```python
from build123d import *

# Parameters (mm, degrees)
F0_W     = 30
F0_H     = 10
F1_DEPTH = 44
F2_R     = 3
F3_R     = 3
F5_START = 44
F4_R     = 2.75
F5_DEPTH = 18
F7_R     = 2.75
F8_ANGLE = 180
F10_W    = 6.5
F10_H    = 4
F12_SIZE = 1
F13_SIZE = 1


with BuildPart() as f1:
    # F0 (on Top) → F1 (new body)
    with BuildSketch(Plane.XY):
        Rectangle(F0_W, F0_H)
    extrude(amount=F1_DEPTH)

    # F2
    f2_edges = [f1.edges().sort_by_distance(p)[0] for p in [
        (15, -5, 22),
        (-15, -5, 22),
    ]]
    fillet(f2_edges, radius=F2_R)

    # F3
    f3_edges = [f1.edges().sort_by_distance(p)[0] for p in [
        (15, 5, 22),
        (-15, 5, 22),
    ]]
    fillet(f3_edges, radius=F3_R)

    # F4 (on Top) → F5 (join)
    with BuildSketch(Plane.XY.offset(F5_START)):
        with Locations((-11, 0)):
            Circle(F4_R)
        with Locations((11, 0)):
            Circle(F4_R)
    extrude(amount=F5_DEPTH)

    # F7 (on offset) → F8 (revolve)
    with BuildSketch(Plane.XY.offset(62)):
        with Locations((11, 0)):
            Circle(F7_R)
    revolve(axis=Axis((0, -1.5820115805, 62), (0, -1, 0)), revolution_arc=F8_ANGLE)

    # F10 (on offset) → F11 (revolve)
    with BuildSketch(Plane.YZ.offset(9)):
        with Locations((-3.25, 23)):
            Rectangle(F10_W, F10_H)
        with Locations((-3.25, 16)):
            Rectangle(F10_W, F10_H)
        with Locations((-3.25, 9)):
            Rectangle(F10_W, F10_H)
    revolve(axis=Axis((9, 0, 12.7572556958), (0, 0, -1)))

    # F12
    f12_edges = [f1.edges().sort_by_distance(p)[0] for p in [
        (15, 0, 44),
        (14.12132, 4.12132, 44),
        (14.12132, -4.12132, 44),
        (-14.12132, 4.12132, 44),
        (-15, 0, 44),
        (-14.12132, -4.12132, 44),
    ]]
    chamfer(f12_edges, length=F12_SIZE)

    # F13
    f13_edges = [f1.edges().sort_by_distance(p)[0] for p in [
        (15, 0, 0),
        (14.12132, 4.12132, 0),
        (14.12132, -4.12132, 0),
        (0, 5, 0),
        (0, -5, 0),
        (-14.12132, 4.12132, 0),
        (-14.12132, -4.12132, 0),
        (-15, 0, 0),
    ]]
    chamfer(f13_edges, length=F13_SIZE)


solid = f1.part
```
The model under review builds one solid part; all positions refer to its coordinate system, in mm. A direction names the side the tool comes from. Coordinates: 2 decimals unless noted, no trailing zeros. Write each loop counter-clockwise with the first axis right and the second up, starting at its lowest first coordinate (ties: lowest second). Pieces come first, ordered by that corner, then holes. Notation, with made-up numbers: (34.25, 75) - (88.25, 75) arc R23 ccw to (88.25, 89) - close; hole circle Ø9 at (13, 73). An arc over 180 degrees is marked (long way). Answer in a Markdown table with one row per item. Add a question column.
Q1. Consider section A-A on y = 0. Give the boundary of the cut face in (x, z).
Q2. To check wall thickness, follow line 1 along Z through (x, y) = (5.5, -4); line 2 along Y through (x, z) = (-7.5, 27.5); line 3 along Z through (x, y) = (6.5, 0.25). State the ranges of each line that lie inside material, in increasing order. Write a range as from..to.
Q3. Clearance check with flat-ended pins moving along their axes: pin 1 (4.5 mm diameter, centred on y = 0.5, z = 4.5, fed in from +X); pin 2 (7 mm diameter, centred on x = -3, z = 13.5, fed in from +Y); pin 3 (5 mm diameter, centred on x = -3, y = -2, fed in from +Z). State where each tip first meets the part, or that it passes through.
Q4. Consider section C-C on z = 22. Give the boundary of the cut face in (x, y).
Q5. For faces 1 (the face through (14.1, -4.14, 22.29)), 2 (the face through (0, 0, 44)), 3 (the face through (15, 0, 4)), list the 3-axis set-ups (+Z, -Z, +X, -X, +Y, -Y) from which the entire face can be reached by the end or side of a thin tool; tool diameter is ignored.
Q6. Draft analysis for pull direction X (two halves, no side actions). For faces 4 (the face through (14.1, 4.14, 22.29)), 5 (the face through (-8.46, -1.05, 52.87)), 6 (the face through (-15, 0, 22)), 7 (the face through (9, -6, 7)), state which applies: +X half, -X half, draft (parallel to the pull), parting line (faces both ways), or undercut.
Q7. Consider section B-B on z = 41. Give the boundary of the cut face in (x, y).
Answers below:
| question | item | result |
|---|---|---|
| 1 | outline | (-15, 1) - (-14, 0) - (14, 0) - (15, 1) - (15, 7) - (15.5, 7) - (15.5, 11) - (15, 11) - (15, 14) - (15.5, 14) - (15.5, 18) - (15, 18) - (15, 21) - (15.5, 21) - (15.5, 25) - (15, 25) - (15, 43) - (14, 44) - (13.75, 44) - (13.75, 62) arc R13.75 ccw to (-13.75, 62) - (-13.75, 44) - (-14, 44) - (-15, 43) - close; hole (-8.25, 44) - (8.25, 44) - (8.25, 62) arc R8.25 ccw to (-8.25, 62) - close |
| 2 | line 1 | 0..44 |
| 2 | line 2 | -5..5 |
| 2 | line 3 | 0..44, 67.1..74.1 |
| 3 | pin 1 | x = 15 |
| 3 | pin 2 | y = 5 |
| 3 | pin 3 | z = 75.68 |
| 4 | outline | (-15, -2) arc R3 ccw to (-12, -5) - (4.85, -5) arc R6.5 ccw to (13.75, -4.44) arc R3 ccw to (14.92, -2.68) arc R6.5 ccw to (14.92, 2.68) arc R3 ccw to (13.75, 4.44) arc R6.5 ccw to (4.85, 5) - (-12, 5) arc R3 ccw to (-15, 2) - close |
| 5 | face 1 | +X, -Y |
| 5 | face 2 | none |
| 5 | face 3 | -Z, +X, +Y, -Y |
| 6 | face 4 | +X half |
| 6 | face 5 | undercut |
| 6 | face 6 | -X half |
| 6 | face 7 | draft |
| 7 | outline | (-15, -2) arc R3 ccw to (-12, -5) - (12, -5) arc R3 ccw to (15, -2) - (15, 2) arc R3 ccw to (12, 5) - (-12, 5) arc R3 ccw to (-15, 2) - close |
